from build123d import *

# Parameters (mm, degrees)
F2_SIZE       = 0.79375
F3_W          = 3.175002
F3_H          = 7.9375
F4_DEPTH      = 12.701
F4_DEPTH_BACK = 12.701
F5_R          = 0.79375


with BuildPart() as f1:
    # F0 (on Front) → F1 (revolve)
    with BuildSketch(Plane.XZ):
        Polygon((12.7, 0), (4.7625, 0), (4.7625, 7.9375), (5.2705, 7.9375), (5.2705, 9.525), (0, 9.525), (0, 7.9375), (0, 0), (0, -1.27), (12.7, -1.27), align=None)
    revolve(axis=Axis((0, 0, 3.96875), (0, 0, 1)))

    # F2
    f2_edges = [f1.edges().sort_by_distance(p)[0] for p in [
        (-5.2705, 0, 9.525),
    ]]
    chamfer(f2_edges, length=F2_SIZE)

    # F3 (on Front) → F4 (cut, two sides)
    with BuildSketch(Plane.XZ) as f4_sk:
        with Locations((0, 5.55625)):
            Rectangle(F3_W, F3_H)
    extrude(amount=F4_DEPTH, mode=Mode.SUBTRACT)
    extrude(f4_sk.sketch, amount=-F4_DEPTH_BACK, mode=Mode.SUBTRACT)

    # F5
    f5_edges = [f1.edges().sort_by_distance(p)[0] for p in [
        (1.587501, 0, 1.5875),
        (-1.587501, 0, 1.5875),
    ]]
    fillet(f5_edges, radius=F5_R)


solid = f1.part
Verification items for the finished model (mm, model axes). A direction names the side the tool comes from. Coordinates: 2 decimals unless noted, no trailing zeros. Order: outer loops, then holes, each group sorted by start corner. A loop starts at its lowest first (then second) coordinate and runs counter-clockwise, first axis right, second up. Notation, with made-up numbers: (50.25, 20.5) -> (99.25, 20.5) arc R10 cw to (99.25, 33.5) -> close; hole circle Ø10 at (51.25, -15). An arc over 180 degrees is marked (long way). Use CSV: the item, a comma, the result in double quotes. Start each with the question number.
Q1. Tool access check on faces 5 (the cylindrical face through (5.27, -0.09, 8.34)), 6 (the flat face through (0, 0, 1.588)), 7 (the flat face through (-5, 0, 7.938)). Record the directions out of +Z, -Z, +X, -X, +Y, -Y that give a thin tool (end or side, any length) a straight path to the whole face; none if there is none.
Q2. Draft check along X on faces 1 (the flat face through (-3, 0, 9.525)), 2 (the flat face through (-1.588, 0, 6)), 3 (the flat face through (1.588, 0, 6)), 4 (the cylindrical face through (-5.27, 0.09, 8.34)). Enter one of: +X half, -X half, draft (parallel to the pull), parting line (faces both ways), or undercut.
Q3. Section check A-A, the plane x = 0. Record the cut outline in (y, z).
Q4. Section check D-D, the plane x = 9.5. Record the cut outline in (y, z), and give its area (3 significant figures).
Q5. Depth check by flat-ended pin: P1, Ø0.8, axis at x = 0, y = -1.5, coming from the +Z side; P2, Ø2, axis at x = -9, z = 0, coming from the -Y side; P3, Ø5.5, axis at y = -0.5, z = 4, coming from the +X side; P4, Ø7.5, axis at x = -1, y = 3, coming from the +Z side (3 decimals). Enter the tip coordinate at first touch or a pass-through.
Q6. Section check B-B, the plane y = 0. Record the cut outline in (x, z) (1 decimal), and give its area (3 significant figures).
Q7. Thickness scan on line 1 along X through (y, z) = (0.75, 3); line 2 along Z through (x, y) = (2.25, 9.5); line 3 along X through (y, z) = (-2.5, 8). Record the ranges inside material, lowest first.
Q8. Section check C-C, the plane z = 1.25. Record the cut outline in (x, y) (1 decimal), and give its area (3 significant figures).
Returned:
1,face 5,"+Z, +X"
1,face 6,"+Z, +Y, -Y"
1,face 7,"-X"
2,face 1,"draft"
2,face 2,"undercut"
2,face 3,"undercut"
2,face 4,"-X half"
3,outline,"(-12.7, -1.27) -> (12.7, -1.27) -> (12.7, 0) -> (4.76, 0) -> (4.76, 1.59) -> (-4.76, 1.59) -> (-4.76, 0) -> (-12.7, 0) -> close"
4,outline,"(-8.43, -1.27) -> (8.43, -1.27) -> (8.43, 0) -> (-8.43, 0) -> close"
4,area,"21.4 mm^2"
5,P1,"stops at z = 1.59"
5,P2,"stops at y = -9.86"
5,P3,"stops at x = 4.76"
5,P4,"stops at z = 9.525"
6,outline,"(-12.7, -1.3) -> (12.7, -1.3) -> (12.7, 0) -> (4.8, 0) -> (4.8, 7.9) -> (5.3, 7.9) -> (5.3, 8.7) -> (4.5, 9.5) -> (1.6, 9.5) -> (1.6, 2.4) arc R0.8 cw to (0.8, 1.6) -> (-0.8, 1.6) arc R0.8 cw to (-1.6, 2.4) -> (-1.6, 9.5) -> (-4.5, 9.5) -> (-5.3, 8.7) -> (-5.3, 7.9) -> (-4.8, 7.9) -> (-4.8, 0) -> (-12.7, 0) -> close"
6,area,"99.0 mm^2"
7,line 1,"x = -4.7 to -1.59, 1.59 to 4.7"
7,line 2,"z = -1.27 to 0"
7,line 3,"x = -4.64 to -1.59, 1.59 to 4.64"
8,outline,"circle Ø9.5 at (0, 0)"
8,area,"71.3 mm^2"
